from build123d import *

# Parameters (mm, degrees)
SKETCH_1_R          = 1.6
EXTRUDE_4_DEPTH     = 13
EXTRUDE_4_2_DEPTH   = 13
EXTRUDE_4_3_DEPTH   = 13
EXTRUDE_4_4_DEPTH   = 13
SKETCH_1_R_2        = 2.1
EXTRUDE_4_5_DEPTH   = 13
EXTRUDE_4_6_DEPTH   = 13
EXTRUDE_4_7_DEPTH   = 13
SKETCH_8_R          = 49
EXTRUDE_5_DEPTH     = 3
SKETCH_9_R          = 2.1
CUT_EXTRUDE_2_DEPTH = 13
SKETCH_3_R          = 8.6
CUT_EXTRUDE_3_DEPTH = 13
SKETCH_6_R          = 4.05
CUT_EXTRUDE_4_DEPTH = 13
CUT_EXTRUDE_5_DEPTH = 13
SKETCH_2_R          = 11.5
CUT_EXTRUDE_6_DEPTH = 13
FILLET_1_R          = 2
CUT_EXTRUDE_7_REACH = 71.361
SKETCH_10_R         = 2.25
EXTRUDE_START       = -3
SKETCH_11_R         = 2.1
EXTRUDE_6_DEPTH     = 3
SKETCH_12_W         = 10
SKETCH_12_H         = 48
EXTRUDE_7_DEPTH     = 10
EXTRUDE_8_DEPTH     = 48
SKETCH_16_W         = 15
SKETCH_16_H         = 4
SKETCH_16_W_2       = 11
SKETCH_16_H_2       = 18.11473671
EXTRUDE_9_DEPTH     = 18
CUT_EXTRUDE_8_DEPTH = 48


with BuildPart() as part:
    # Sketch 1 → Extrude 4 (new body)
    with BuildSketch(Plane.XY):
        with Locations((0, 44)):
            Circle(SKETCH_1_R)
    extrude(amount=EXTRUDE_4_DEPTH)



with BuildPart() as body_2:
    # Sketch 1 → Extrude 4 2 (new body)
    with BuildSketch(Plane.XY):
        with Locations((44, 0)):
            Circle(SKETCH_1_R)
    extrude(amount=EXTRUDE_4_2_DEPTH)


with BuildPart() as body_3:
    # Sketch 1 → Extrude 4 3 (new body)
    with BuildSketch(Plane.XY):
        with Locations((0, -44)):
            Circle(SKETCH_1_R)
    extrude(amount=EXTRUDE_4_3_DEPTH)


with BuildPart() as body_4:
    # Sketch 1 → Extrude 4 4 (new body)
    with BuildSketch(Plane.XY):
        with Locations((-44, 0)):
            Circle(SKETCH_1_R)
    extrude(amount=EXTRUDE_4_4_DEPTH)


with BuildPart() as body_5:
    # Sketch 1 → Extrude 4 5 (new body)
    with BuildSketch(Plane.XY):
        with Locations((29, 0)):
            Circle(SKETCH_1_R_2)
    extrude(amount=EXTRUDE_4_5_DEPTH)


with BuildPart() as body_6:
    # Sketch 1 → Extrude 4 6 (new body)
    with BuildSketch(Plane.XY):
        with Locations((-14.5, 25.11473671)):
            Circle(SKETCH_1_R_2)
    extrude(amount=EXTRUDE_4_6_DEPTH)


with BuildPart() as body_7:
    # Sketch 1 → Extrude 4 7 (new body)
    with BuildSketch(Plane.XY):
        with Locations((-14.5, -25.11473671)):
            Circle(SKETCH_1_R_2)
    extrude(amount=EXTRUDE_4_7_DEPTH)


with BuildPart() as part_1:
    add(part.part)

    add(body_2.part)  # Extrude 5 merges body 2

    add(body_3.part)  # Extrude 5 merges body 3

    add(body_4.part)  # Extrude 5 merges body 4

    add(body_5.part)  # Extrude 5 merges body 5

    add(body_6.part)  # Extrude 5 merges body 6

    add(body_7.part)  # Extrude 5 merges body 7
    # Sketch 8 → Extrude 5 (add)
    with BuildSketch(Plane.XY):
        Circle(SKETCH_8_R)
    extrude(amount=EXTRUDE_5_DEPTH)

    # Sketch 9 → Cut-Extrude 2 (cut)
    with BuildSketch(Plane.XY):
        with Locations((0, 44)):
            Circle(SKETCH_9_R)
        with Locations((44, 0)):
            Circle(SKETCH_9_R)
        with Locations((0, -44)):
            Circle(SKETCH_9_R)
        with Locations((-44, 0)):
            Circle(SKETCH_9_R)
        with Locations((-14.5, 25.11473671)):
            Circle(SKETCH_9_R)
        with Locations((-14.5, -25.11473671)):
            Circle(SKETCH_9_R)
        with Locations((29, 0)):
            Circle(SKETCH_9_R)
    extrude(amount=CUT_EXTRUDE_2_DEPTH, mode=Mode.SUBTRACT)

    # Sketch 3 → Cut-Extrude 3 (cut)
    with BuildSketch(Plane.XY):
        Circle(SKETCH_3_R)
    extrude(amount=CUT_EXTRUDE_3_DEPTH, mode=Mode.SUBTRACT)

    # Sketch 6 → Cut-Extrude 4 (cut)
    with BuildSketch(Plane.XY):
        with Locations((19.25, 0)):
            Circle(SKETCH_6_R)
    extrude(amount=CUT_EXTRUDE_4_DEPTH, mode=Mode.SUBTRACT)

    # Sketch 7 → Cut-Extrude 5 (cut)
    with BuildSketch(Plane.XY):
        Polygon((10.802199699, 10.505830841), (14.272482459, 16.5145615), (7.171657827, 20.615572296), (3.701375067, 14.606841637), align=None)
    extrude(amount=CUT_EXTRUDE_5_DEPTH, mode=Mode.SUBTRACT)

    # Sketch 2 → Cut-Extrude 6 (cut)
    with BuildSketch(Plane.XY):
        Circle(SKETCH_2_R)
    extrude(amount=CUT_EXTRUDE_6_DEPTH, mode=Mode.SUBTRACT)

    # Fillet 1
    fillet_1_edges = [part_1.edges().sort_by_distance(p)[0] for p in [
        (7.171657827, 20.615572296, 1.5),
        (3.701375067, 14.606841637, 1.5),
        (10.802199699, 10.505830841, 1.5),
        (14.272482459, 16.5145615, 1.5),
    ]]
    fillet(fillet_1_edges, radius=FILLET_1_R)

    # Sketch 10 → Cut-Extrude 7 (cut, up to next)
    with BuildSketch(Plane.XY.offset(3), mode=Mode.PRIVATE) as cut_extrude_7_sk1:
        with Locations((-31.112698372, 31.112698372)):
            Circle(SKETCH_10_R)
    cut_extrude_7_tool1 = extrude(cut_extrude_7_sk1.sketch, amount=-CUT_EXTRUDE_7_REACH, mode=Mode.PRIVATE) & part_1.part
    # Sketch 10 → Cut-Extrude 7 (cut, up to next)
    with BuildSketch(Plane.XY.offset(3), mode=Mode.PRIVATE) as cut_extrude_7_sk2:
        with Locations((31.112698372, 31.112698372)):
            Circle(SKETCH_10_R)
    cut_extrude_7_tool2 = extrude(cut_extrude_7_sk2.sketch, amount=-CUT_EXTRUDE_7_REACH, mode=Mode.PRIVATE) & part_1.part
    # Sketch 10 → Cut-Extrude 7 (cut, up to next)
    with BuildSketch(Plane.XY.offset(3), mode=Mode.PRIVATE) as cut_extrude_7_sk3:
        with Locations((31.112698372, -31.112698372)):
            Circle(SKETCH_10_R)
    cut_extrude_7_tool3 = extrude(cut_extrude_7_sk3.sketch, amount=-CUT_EXTRUDE_7_REACH, mode=Mode.PRIVATE) & part_1.part
    # Sketch 10 → Cut-Extrude 7 (cut, up to next)
    with BuildSketch(Plane.XY.offset(3), mode=Mode.PRIVATE) as cut_extrude_7_sk4:
        with Locations((-31.112698372, -31.112698372)):
            Circle(SKETCH_10_R)
    cut_extrude_7_tool4 = extrude(cut_extrude_7_sk4.sketch, amount=-CUT_EXTRUDE_7_REACH, mode=Mode.PRIVATE) & part_1.part
    add(cut_extrude_7_tool1.solids().sort_by_distance((-31.112698, 31.112698, 3))[0], mode=Mode.SUBTRACT)
    add(cut_extrude_7_tool2.solids().sort_by_distance((31.112698, 31.112698, 3))[0], mode=Mode.SUBTRACT)
    add(cut_extrude_7_tool3.solids().sort_by_distance((31.112698, -31.112698, 3))[0], mode=Mode.SUBTRACT)
    add(cut_extrude_7_tool4.solids().sort_by_distance((-31.112698, -31.112698, 3))[0], mode=Mode.SUBTRACT)

    # Sketch 11 → Extrude 6 (add)
    with BuildSketch(Plane.XY.offset(3).offset(EXTRUDE_START)):
        with Locations((-44, 0)):
            Circle(SKETCH_11_R)
        with Locations((0, -44)):
            Circle(SKETCH_11_R)
        with Locations((44, 0)):
            Circle(SKETCH_11_R)
        with Locations((0, 44)):
            Circle(SKETCH_11_R)
    extrude(amount=EXTRUDE_6_DEPTH)

    # Sketch 12 → Extrude 7 (add)
    with BuildSketch(Plane(origin=(0, 0, 0), x_dir=(-1, 0, 0), z_dir=(0, 0, -1))):
        with Locations((31, 0)):
            Rectangle(SKETCH_12_W, SKETCH_12_H)
    extrude(amount=EXTRUDE_7_DEPTH)

    # Sketch 13 → Extrude 8 (add)
    with BuildSketch(Plane(origin=(0, 24, 0), x_dir=(1, 0, 0), z_dir=(0, 1, 0))):
        Polygon((0, 20.784609691), (-26, 5.773502692), (-26, 2.309401077), (0, 17.320508076), align=None)
        Polygon((-26, 5.773502692), (-36, 0), (-30, 0), (-26, 2.309401077), align=None)
    extrude(amount=-EXTRUDE_8_DEPTH)

    # Sketch 16 → Extrude 9 (add)
    with BuildSketch(Plane(origin=(0, 0, 0), x_dir=(-1, 0, 0), z_dir=(0, 0, -1))):
        with Locations((7.5, -20.11473671)):
            Rectangle(SKETCH_16_W, SKETCH_16_H)
        with Locations((20.5, -20.11473671)):
            Rectangle(SKETCH_16_W_2, SKETCH_16_H)
        with Locations((20.5, -9.057368355)):
            Rectangle(SKETCH_16_W_2, SKETCH_16_H_2)
        with Locations((7.5, 20.11473671)):
            Rectangle(SKETCH_16_W, SKETCH_16_H)
        with Locations((20.5, 20.11473671)):
            Rectangle(SKETCH_16_W_2, SKETCH_16_H)
        with Locations((20.5, 9.057368355)):
            Rectangle(SKETCH_16_W_2, SKETCH_16_H_2)
    extrude(amount=EXTRUDE_9_DEPTH)

    # Sketch 14 → Cut-Extrude 8 (cut)
    with BuildSketch(Plane(origin=(0, 24, 0), x_dir=(1, 0, 0), z_dir=(0, 1, 0))):
        Polygon((0, 20.784609691), (-36, 20.784609691), (-36, 0), align=None)
    extrude(amount=-CUT_EXTRUDE_8_DEPTH, mode=Mode.SUBTRACT)


solid = part_1.part
The model under review builds one solid part; all positions refer to its coordinate system, in mm. A direction names the side the tool comes from. Coordinates: 2 decimals unless noted, no trailing zeros. Loops run counter-clockwise (first coordinate to the right, second up) from the corner with the lowest first, then second, coordinate; pieces in that order, holes last.
(1) Consider section C-C, the plane z = -4.5. Give the boundary of the cut face in (x, y), plus the area to 3 significant figures.
Determined:
outline: (-28.21, -24) - (-22.21, -24) - (-22.21, -22.11) - (0, -22.11) - (0, -18.11) - (-15, -18.11) - (-15, 18.11) - (0, 18.11) - (0, 22.11) - (-22.21, 22.11) - (-22.21, 24) - (-28.21, 24) - close
area: 727 mm2
(2) Consider section B-B, the plane y = 0. Give the boundary of the cut face in (x, z).
Determined:
outline: (-49, 0) - (-36, 0) - (0, -20.78) - (0, -17.32) - (-15, -8.66) - (-15, 0) - (-11.5, 0) - (-11.5, 3) - (-49, 3) - close; (11.5, 0) - (15.2, 0) - (15.2, 3) - (11.5, 3) - close; (23.3, 0) - (26.9, 0) - (26.9, 3) - (23.3, 3) - close; (31.1, 0) - (49, 0) - (49, 3) - (31.1, 3) - close
(3) Tool access review of faces 1 (the flat face through (-13.2, 23.1, -9.7)), 2 (the flat face through (-13.2, -23, -9.7)), 3 (the cylindrical face through (-13.371, 26.885, 1.479)): name each direction out of +Z, -Z, +X, -X, +Y, -Y from which nothing blocks a thin tool from reaching the whole face with its end or side.
Determined:
face 1: +X, +Y
face 2: +X, -Y
face 3: +Z
(4) Consider section D-D, the plane y = 36. Give the boundary of the cut face in (x, z), plus the area to 3 significant figures.
Determined:
outline: (-33.24, 0) - (33.24, 0) - (33.24, 3) - (-33.24, 3) - close
area: 199 mm2
(5) Draft analysis for pull direction Z (two halves, no side actions). For faces 4 (the flat face through (-12, 1, 3)), 5 (the flat face through (-10, 22.115, -7)), 6 (the flat face through (12.527, 13.492, 1.479)), state which applies: +Z half, -Z half, draft (parallel to the pull), parting line (faces both ways), or undercut.
Determined:
face 4: +Z half
face 5: undercut
face 6: draft
(6) Insertion check: P1, Ø6, axis at y = 31, z = 0, coming from the +X side; P2, Ø3, axis at x = 31.5, z = -0.5, coming from the +Y side; P3, Ø7.5, axis at x = -9, z = -9.5, coming from the +Y side; P4, Ø12, axis at x = 37.5, z = -6.5, coming from the +Y side. Each pin has a flat end and moves straight along its axis. Give the tip position at first contact, or say it passes through.
Determined:
P1: stops at x = 40.21
P2: stops at y = 38.68
P3: stops at y = 24
P4: passes through
(7) Wall thickness on L1, parallel to Y at x = -10.5, z = -3.5; L2, parallel to Y at x = -10.5, z = -14.25; L3, parallel to Z at x = 1, y = 21: over which ranges is each line inside the solid? List them lowest first.
Determined:
L1: y = -22.11 to -18.11, 18.11 to 22.11
L2: y = -24 to 24
L3: z = 0 to 3
(8) Consider section A-A, the plane x = 19. Give the boundary of the cut face in (y, z), plus the area to 3 significant figures.
Determined:
outline: (-45.17, 0) - (-4.04, 0) - (-4.04, 3) - (-45.17, 3) - close; (4.04, 0) - (45.17, 0) - (45.17, 3) - (4.04, 3) - close
area: 247 mm2
